```python
from build123d import *

# Parameters (mm, degrees)
SKETCH1_W           = 100
SKETCH1_H           = 100
SKETCH1_R           = 8
BOSS_EXTRUDE1_DEPTH = 15
SKETCH4_W           = 15
SKETCH4_H           = 30
BOSS_EXTRUDE2_DEPTH = 10
SKETCH7_W           = 15
SKETCH7_H           = 30
BOSS_EXTRUDE3_DEPTH = 10
SKETCH8_R           = 15
CUT_EXTRUDE1_DEPTH  = 5
CUT_EXTRUDE2_START  = -5
SKETCH10_R          = 15
CUT_EXTRUDE2_DEPTH  = 5
SKETCH11_R          = 12.5
CUT_EXTRUDE5_DEPTH  = 150.415527975
SKETCH12_R          = 4
CUT_EXTRUDE6_DEPTH  = 20
CUT_EXTRUDE7_START  = -20
SKETCH13_R          = 4
CUT_EXTRUDE7_DEPTH  = 20


with BuildPart() as part:
    # Sketch1 → Boss-Extrude1 (new body)
    with BuildSketch(Plane.XY):
        with Locations((50, 50)):
            Rectangle(SKETCH1_W, SKETCH1_H)
        with Locations((15, 85)):
            Circle(SKETCH1_R, mode=Mode.SUBTRACT)
        with Locations((85, 85)):
            Circle(SKETCH1_R, mode=Mode.SUBTRACT)
        with Locations((85, 15)):
            Circle(SKETCH1_R, mode=Mode.SUBTRACT)
        with Locations((15, 15)):
            Circle(SKETCH1_R, mode=Mode.SUBTRACT)
    extrude(amount=BOSS_EXTRUDE1_DEPTH)

    # Sketch4 → Boss-Extrude2 (add)
    with BuildSketch(Plane(origin=(100, 0, 0), x_dir=(0, 0, -1), z_dir=(1, 0, 0))):
        with Locations((-7.5, 50)):
            Rectangle(SKETCH4_W, SKETCH4_H)
    extrude(amount=BOSS_EXTRUDE2_DEPTH)

    # Sketch7 → Boss-Extrude3 (add)
    with BuildSketch(Plane.ZY):
        with Locations((7.5, 50)):
            Rectangle(SKETCH7_W, SKETCH7_H)
    extrude(amount=BOSS_EXTRUDE3_DEPTH)

    # Sketch8 → Cut-Extrude1 (cut)
    with BuildSketch(Plane.XY.offset(15)):
        with Locations((50, 50)):
            Circle(SKETCH8_R)
    extrude(amount=-CUT_EXTRUDE1_DEPTH, mode=Mode.SUBTRACT)

    # Sketch10 → Cut-Extrude2 (cut)
    with BuildSketch(Plane(origin=(0, 0, 0), x_dir=(-1, 0, 0), z_dir=(0, 0, -1)).offset(CUT_EXTRUDE2_START)):
        with Locations(Location((-50, 50, 0), (0, 0, 180))):
            Circle(SKETCH10_R)
    extrude(amount=CUT_EXTRUDE2_DEPTH, mode=Mode.SUBTRACT)

    # Sketch11 → Cut-Extrude5 (cut, through all)
    with BuildSketch(Plane(origin=(0, 0, 0), x_dir=(-1, 0, 0), z_dir=(0, 0, -1))):
        with Locations((-50, 50)):
            Circle(SKETCH11_R)
    extrude(amount=-CUT_EXTRUDE5_DEPTH, mode=Mode.SUBTRACT)

    # Sketch12 → Cut-Extrude6 (cut)
    with BuildSketch(Plane(origin=(110, 0, 0), x_dir=(0, 0, -1), z_dir=(1, 0, 0))):
        with Locations((-7.5, 50)):
            Circle(SKETCH12_R)
    extrude(amount=-CUT_EXTRUDE6_DEPTH, mode=Mode.SUBTRACT)

    # Sketch13 → Cut-Extrude7 (cut)
    with BuildSketch(Plane.ZY.offset(10).offset(CUT_EXTRUDE7_START)):
        with Locations(Location((7.5, 50, 0), (0, 0, 180))):
            Circle(SKETCH13_R)
    extrude(amount=CUT_EXTRUDE7_DEPTH, mode=Mode.SUBTRACT)


solid = part.part
```
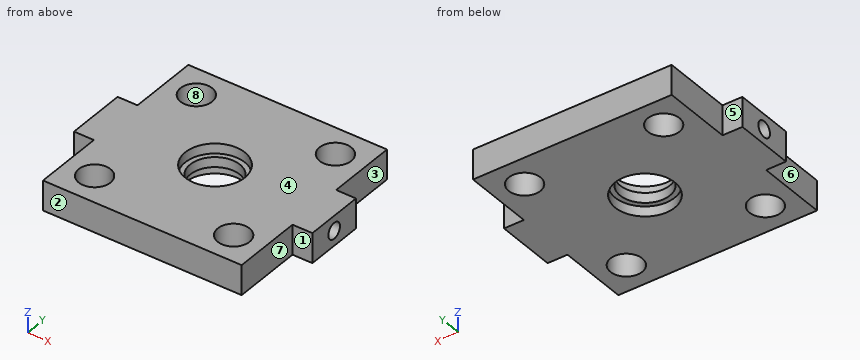
Can you work these out from the model? Positions are in its coordinate system, mm. Face numbers are marked on the shaded views. A direction names the side the tool comes from. Coordinates: 2 decimals unless noted, no trailing zeros. Write each loop counter-clockwise with the first axis right and the second up, starting at its lowest first coordinate (ties: lowest second). Pieces come first, ordered by that corner, then holes. Notation, with made-up numbers: M 62.5,-36 L 103.5,-36 A10 cw 103.5,-24 Z; hole C 73.25,-20.75 d11. An arc over 180 degrees is marked long. Write item = value, one per line. Start each with the question number.
Q1. If we section it at B-B, the plane x = 50: Write out the boundary of the cut face in (y, z), then the cut area to 4 significant figures.
Q2. Thinking about a two-plate mould opening in X: for the marked faces 6, 7 and 8, which applies, released by +X, released by -X, zero draft, split by the parting line, or undercut?
Q3. If I drill on L1, parallel to Y at x = 15, z = 8.25; L2, parallel to X at y = 9.5, z = 7.5; L3, parallel to Y at x = 101.5, z = 7.5, over which ranges is the centre line in solid material (lowest first)? Write a range as [from, to].
Q4. On a 3-axis mill with a long thin cutter (end or side, diameter ignored), from which of +Z, -Z, +X, -X, +Y, -Y can I reach the whole of each face in a straight line? I mean the marked faces 1, 2, 3, 4 and 5. Say none if no direction works.
Q5. If we section it at C-C, the plane z = 7.5: Write out the boundary of the cut face in (x, y).
Q6. I'm going to push flat-ended pins straight in: pin 1 (3 mm diameter, centred on y = 19, z = 7, fed in from +X); pin 2 (5 mm diameter, centred on x = 103, z = 5.5, fed in from -Y); pin 3 (3 mm diameter, centred on x = -7, z = 4, fed in from +Y). Where does each tip first touch, or does it pass through?
Q7. If we section it at A-A, the plane y = 85: Write out the boundary of the cut face in (x, z), then the cut area to 3 significant figures.
Check sheet entries:
q1.outline = M 0,0 L 35,0 L 35,5 L 37.5,5 L 37.5,10 L 35,10 L 35,15 L 0,15 Z; M 62.5,5 L 65,5 L 65,0 L 100,0 L 100,15 L 65,15 L 65,10 L 62.5,10 Z
q1.area = 1,075 mm²
q2.face_6 = released by -X
q2.face_7 = released by +X
q2.face_8 = undercut
q3.L1 = [0, 7], [23, 77], [93, 100]
q3.L2 = [0, 9.19], [20.81, 79.19], [90.81, 100]
q3.L3 = [35, 46], [54, 65]
q4.face_1 = +Z, -Z, +X, -Y
q4.face_2 = +Z, -Z, +X, -X, -Y
q4.face_3 = +Z, -Z, +X, +Y
q4.face_4 = +Z, +X, -X, +Y, -Y
q4.face_5 = +Z, -Z, -X, +Y
q5.outline = M -10,35 L 0,35 L 0,0 L 100,0 L 100,35 L 110,35 L 110,46 L 90,46 L 90,54 L 110,54 L 110,65 L 100,65 L 100,100 L 0,100 L 0,65 L -10,65 L -10,54 L 10,54 L 10,46 L -10,46 Z; hole C 15,15 d16; hole C 15,85 d16; hole C 50,50 d25; hole C 85,15 d16; hole C 85,85 d16
q6.pin_1 = 100
q6.pin_2 = 35
q6.pin_3 = 65
q7.outline = M 0,0 L 7,0 L 7,15 L 0,15 Z; M 23,0 L 77,0 L 77,15 L 23,15 Z; M 93,0 L 100,0 L 100,15 L 93,15 Z
q7.area = 1,020 mm²
